Verification items for the finished model (mm, model axes). A direction names the side the tool comes from. Give positions to 0.01 mm unless a question says otherwise; leave off trailing zeros. Order: outer loops, then holes, each group sorted by start corner. A loop starts at its lowest first (then second) coordinate and runs counter-clockwise, first axis right, second up.
(1) Scan lines: L1, parallel to Y at x = -128, z = 0.45; L2, parallel to Y at x = -75, z = -0.3; L3, parallel to Y at x = -30, z = -0.6. Record each from-to range of solid material in increasing order.
(2) Mould release check, pull along Y, two halves, no side actions. Record for faces 4 (the face through (-31.493, 0.154, -0.021)), 5 (the face through (-136.955, -17.376, 0.021)), 6 (the face through (-112.5, -13, 0)): pulls with the +Y half, pulls with the -Y half, needs draft (parallel to the pull), parting line crosses it, or undercut.
(3) Sectioned sample at A-A on y = 9. Record the cut outline in (x, z), plus the area to 3 significant figures.
(4) Sectioned sample at B-B on x = -125.5. Count the separate pieces of the cut face and the enclosed holes in it, plus the area to 3 significant figures.
(5) Access from +Z, -Z, +X, -X, +Y, -Y to the whole of each face (thin tool, end or side, straight path). Record for faces 1 (the face through (-53, -17.5, 0)), 2 (the face through (-140.292, 0.742, 0.021)), 3 (the face through (-114.413, -11, 0)).
(6) Sectioned sample at D-D on x = -101.5. Record the cut outline in (y, z).
(7) Gauge pin test, flat ends, axial feed: pin 1 (2 mm diameter, centred on x = -108.5, y = -7, fed in from +Z); pin 2 (0.9 mm diameter, centred on x = -56.5, z = -0.5, fed in from -Y); pin 3 (4 mm diameter, centred on x = -28, y = 0, fed in from +Z); pin 4 (1.5 mm diameter, centred on x = -61.5, z = -0.5, fed in from +Y). Record the tip position at first contact, or that the pin passes through.
(8) Sectioned sample at C-C on y = -8.5. Record the cut outline in (x, z).
```python
from build123d import *

# Parameters (mm, degrees)
F0_R     = 3.5
F1_DEPTH = 1.5


# Not quite as in the source:
# - a feature names something its author has since deleted; it is built from what else it names


with BuildPart() as f1:
    # F0 (on Top) → F1 (new body, symmetric)
    with BuildSketch(Plane.XY):
        with BuildLine():
            Line((-140.2163859753, 11.480502971), (-117.1193976626, 1.9134171618))
            ThreePointArc((-117.1193976626, 1.9134171618), (-117.2054191616, 1.6908667936), (-117.2807257879, 1.4644660941))
            Line((-117.2807257879, 1.4644660941), (-135.5639451435, 1.4644660941))
            Line((-135.5639451435, 1.4644660941), (-137.4212426417, 1.4644660941))
            Line((-137.4212426417, 1.4644660941), (-137.4642343313, 1.4644660941))
            Line((-137.4642343313, 1.4644660941), (-143.2, 0))
            Line((-143.2, 0), (-137.4642343313, -1.4644660941))
            Line((-137.4642343313, -1.4644660941), (-137.4212426417, -1.4644660941))
            Line((-137.4212426417, -1.4644660941), (-135.5639451435, -1.4644660941))
            Line((-135.5639451435, -1.4644660941), (-117.2807257879, -1.4644660941))
            ThreePointArc((-117.2807257879, -1.4644660941), (-117.2054191616, -1.6908667936), (-117.1193976626, -1.9134171618))
            Line((-117.1193976626, -1.9134171618), (-140.2163859753, -11.480502971))
            ThreePointArc((-140.2163859753, -11.480502971), (-137.4440883691, -16.6671069906), (-133.7132034356, -21.2132034356))
            ThreePointArc((-133.7132034356, -21.2132034356), (-133.0255631487, -21.8792426155), (-132.3170219693, -22.5230024701))
            add(Edge.make_bspline(
                [(-132.3170219693, -22.5230024701), (-131.8310141521, -22.9279318204), (-131.3450063349, -23.3328611708), (-130.8554027807, -23.7292896809)],
                knots=[0, 0, 0, 0, 0.0899480821, 0.0899480821, 0.0899480821, 0.0899480821], degree=3))
            add(Edge.make_bspline(
                [(-130.8554027807, -23.7292896809), (-128.7296529668, -25.4504941622), (-123.6181233569, -29.0879440293), (-116.5404183436, -28.0770720452), (-112.5, -27.5)],
                knots=[0.0899480821, 0.0899480821, 0.0899480821, 0.0899480821, 0.4804826627, 1, 1, 1, 1], degree=3))
            ThreePointArc((-112.5, -27.5), (-122.1329967473, -25.7576274852), (-130.5453194023, -20.7512999031))
            Line((-130.5453194023, -20.7512999031), (-127.2940194993, -17.5))
            Line((-127.2940194993, -17.5), (-114.4134171618, -4.6193976626))
            Line((-114.4134171618, -4.6193976626), (-114.4134171618, -17.6193976626))
            add(Edge.make_bspline(
                [(-114.4134171618, -17.6193976626), (-114.1696893018, -17.7059100784), (-113.5209993488, -17.936165803), (-112.89241231, -19.2067830939), (-112.5, -20)],
                knots=[0, 0, 0, 0, 0.3757231924, 1, 1, 1, 1], degree=3))
            Line((-112.5, -20), (-112.5, -5))
            Line((-112.5, -5), (-77.9963913669, -17.5))
            Line((-77.9963913669, -17.5), (-27.9963913669, -17.5))
            ThreePointArc((-27.9963913669, -17.5), (-10.4963913669, 0), (-27.9963913669, 17.5))
            Line((-27.9963913669, 17.5), (-77.9963913669, 17.5))
            Line((-77.9963913669, 17.5), (-112.5, 5))
            Line((-112.5, 5), (-112.5, 20))
            add(Edge.make_bspline(
                [(-114.4134171618, 17.6193976626), (-114.1696893018, 17.7059100784), (-113.5209993488, 17.936165803), (-112.89241231, 19.2067830939), (-112.5, 20)],
                knots=[0, 0, 0, 0, 0.3757231924, 1, 1, 1, 1], degree=3))
            Line((-114.4134171618, 17.6193976626), (-114.4134171618, 4.6193976626))
            Line((-114.4134171618, 4.6193976626), (-127.2940194993, 17.5))
            Line((-127.2940194993, 17.5), (-130.5453194023, 20.7512999031))
            ThreePointArc((-130.5453194023, 20.7512999031), (-122.1329967473, 25.7576274852), (-112.5, 27.5))
            add(Edge.make_bspline(
                [(-132.3170219693, 22.5230024701), (-129.7208762292, 24.6860450606), (-124.3176724473, 29.1878570062), (-116.5404183436, 28.0770720452), (-112.5, 27.5)],
                knots=[0, 0, 0, 0, 0.4804826627, 1, 1, 1, 1], degree=3))
            Line((-132.3170219693, 22.5230024701), (-133.7132034356, 21.2132034356))
            ThreePointArc((-133.7132034356, 21.2132034356), (-137.4440883691, 16.6671069906), (-140.2163859753, 11.480502971))
        make_face()
        with Locations((-27.9963913669, 0)):
            Circle(F0_R, mode=Mode.SUBTRACT)
    extrude(amount=F1_DEPTH, both=True)


solid = f1.part
```
Ans:
1. L1: y = -25.84 to -22.72, -18.21 to -6.42, -1.46 to 1.46, 6.42 to 18.21, 22.72 to 25.84
1. L2: y = -17.5 to 17.5
1. L3: y = -17.5 to -2.87, 2.87 to 17.5
2. face 4: undercut
2. face 5: pulls with the -Y half
2. face 6: needs draft
3. outline: (-134.23, -1.5) - (-118.79, -1.5) - (-118.79, 1.5) - (-134.23, 1.5) - close; (-114.41, -1.5) - (-112.5, -1.5) - (-112.5, 1.5) - (-114.41, 1.5) - close; (-101.46, -1.5) - (-12.99, -1.5) - (-12.99, 1.5) - (-101.46, 1.5) - close
3. area: 317 mm2
4. separate pieces: 5
4. enclosed holes: 0
4. area: 88.4 mm2
5. face 1: +Z, -Z, +X, -Y
5. face 2: +Z, -Z, -X
5. face 3: +Z, -Z
6. outline: (-8.99, -1.5) - (8.99, -1.5) - (8.99, 1.5) - (-8.99, 1.5) - close
7. pin 1: stops at z = 1.5
7. pin 2: stops at y = -17.5
7. pin 3: passes through
7. pin 4: stops at y = 17.5
8. outline: (-133.02, -1.5) - (-118.29, -1.5) - (-118.29, 1.5) - (-133.02, 1.5) - close; (-114.41, -1.5) - (-112.5, -1.5) - (-112.5, 1.5) - (-114.41, 1.5) - close; (-102.84, -1.5) - (-12.7, -1.5) - (-12.7, 1.5) - (-102.84, 1.5) - close
